from build123d import *

# Parameters (mm, degrees)
SWEEP1_START       = -3.175
SWEEP1_OUTLINE_W   = 31.75
SWEEP1_OUTLINE_H   = 57.15
SWEEP1_OUTLINE_W_2 = 19.05
SWEEP1_OUTLINE_H_2 = 44.45
SWEEP1_DEPTH       = 6.35
FILLET1_R          = 10
FILLET2_R          = 10


# Read off the part's stored shape, not the designer's step: Sweep1
with BuildPart() as part:
    # Sweep1 outline → Sweep1 (new body)
    with BuildSketch(Plane.XY.offset(SWEEP1_START)):
        with Locations((12.7, 25.4)):
            Rectangle(SWEEP1_OUTLINE_W, SWEEP1_OUTLINE_H)
        with Locations((12.7, 25.4)):
            Rectangle(SWEEP1_OUTLINE_W_2, SWEEP1_OUTLINE_H_2, mode=Mode.SUBTRACT)
    extrude(amount=SWEEP1_DEPTH)

    # Fillet1
    # the kernel refuses this fillet: 10 mm, written as the material it adds along each edge
    with BuildSketch(Plane(origin=(3.175, 3.175, -3.175), x_dir=(1, 0, 0), z_dir=(0, 0, 1)), Plane(origin=(22.225, 3.175, -3.175), x_dir=(0, 1, 0), z_dir=(0, 0, 1)), Plane(origin=(22.225, 47.625, -3.175), x_dir=(-1, 0, 0), z_dir=(0, 0, 1))) as fillet1_piece_1:
        with BuildLine():
            CenterArc((FILLET1_R, FILLET1_R), FILLET1_R, 180, 90)
            Line((0, FILLET1_R), (0, 0))
            Line((0, 0), (FILLET1_R, 0))
        make_face()
    extrude(amount=6.35)
    with BuildSketch(Plane(origin=(3.175, 47.625, -3.175), x_dir=(1, 0, 0), z_dir=(0, 0, 1))) as fillet1_piece_2:
        with BuildLine():
            CenterArc((FILLET1_R, -FILLET1_R), FILLET1_R, 90, 90)
            Line((0, -FILLET1_R), (0, 0))
            Line((0, 0), (FILLET1_R, 0))
        make_face()
    extrude(amount=6.35)

    # Fillet2
    fillet2_edges = [part.edges().sort_by_distance(p)[0] for p in [
        (28.575, -3.175, 0),
        (-3.175, 53.975, 0),
        (-3.175, -3.175, 0),
        (28.575, 53.975, 0),
    ]]
    fillet(fillet2_edges, radius=FILLET2_R)


solid = part.part
The model under review builds one solid part; all positions refer to its coordinate system, in mm. A direction names the side the tool comes from. Give positions to 0.01 mm unless a question says otherwise; leave off trailing zeros. Order: outer loops, then holes, each group sorted by start corner. A loop starts at its lowest first (then second) coordinate and runs counter-clockwise, first axis right, second up. Notation, with made-up numbers: M 46,-23 L 77,-23 A31 ccw 77,4 Z; hole C 89,23.25 d2. An arc over 180 degrees is marked long. Use one line per item in the form item = value. Start each with the question number.
Item 1: We need section D-D on y = 1. Give the boundary of the cut face in (x, z) (3 decimals), plus the area to 3 significant figures.
Item 2: We need section B-B on x = 14.5. Give the boundary of the cut face in (y, z) (3 decimals).
Item 3: The part is to be moulded in two halves that separate along Y. For faces 1 (the flat face through (22.225, 25, 0)), 2 (the cylindrical face through (25.57, -0.32, 0.04)), 3 (the flat face through (24, 26, 3.175)), say which applies: pulls with the +Y half, pulls with the -Y half, needs draft (parallel to the pull), parting line crosses it, or undercut.
Item 4: Insertion check: pin 1 Ø2 at (x, z) = (1, -2.5) entering from -Y. The pin has a flat end and moves straight along its axis. Give the tip position at first contact, or say it passes through.
Item 5: We need section C-C on z = 1. Give the boundary of the cut face in (x, y) (3 decimals), plus the area to 3 significant figures.
Item 6: To check wall thickness, follow line 1 along X through (y, z) = (19.5, 0.25) (3 decimals); line 2 along X through (y, z) = (5.5, 2.25); line 3 along Y through (x, z) = (8, 1.75) (3 decimals). State the ranges of each line that lie inside material, in increasing order. Write a range as from..to.
Item 7: For faces 4 (the cylindrical face through (25.57, 51.12, 0.04)), 5 (the cylindrical face through (5.865, 6.351, -0.044)), list the 3-axis set-ups (+Z, -Z, +X, -X, +Y, -Y) from which the entire face can be reached by the end or side of a thin tool; tool diameter is ignored.
Item 8: We need section A-A on y = 33. Give the boundary of the cut face in (x, z) (3 decimals), plus the area to 3 significant figures.
Completed:
q1.outline = M -1.303,-3.175 L 26.703,-3.175 L 26.703,3.175 L -1.303,3.175 Z
q1.area = 178 mm²
q2.outline = M -3.175,-3.175 L 3.437,-3.175 L 3.437,3.175 L -3.175,3.175 Z; M 47.363,-3.175 L 53.975,-3.175 L 53.975,3.175 L 47.363,3.175 Z
q3.face_1 = undercut
q3.face_2 = pulls with the -Y half
q3.face_3 = needs draft
q4.pin_1 = -1.93
q5.outline = M -3.175,6.825 A10 ccw 6.825,-3.175 L 18.575,-3.175 A10 ccw 28.575,6.825 L 28.575,43.975 A10 ccw 18.575,53.975 L 6.825,53.975 A10 ccw -3.175,43.975 Z; hole M 3.175,13.175 A10 ccw 12.7,3.186 A10 ccw 22.225,13.175 L 22.225,37.625 A10 ccw 12.7,47.614 A10 ccw 3.175,37.625 Z
q5.area = 968 mm²
q6.line_1 = -3.175..3.175, 22.225..28.575
q6.line_2 = -3.09..6.76, 18.64..28.49
q6.line_3 = -3.175..4.618, 46.182..53.975
q7.face_4 = +Z, -Z, +X, +Y
q7.face_5 = +Z, -Z
q8.outline = M -3.175,-3.175 L 3.175,-3.175 L 3.175,3.175 L -3.175,3.175 Z; M 22.225,-3.175 L 28.575,-3.175 L 28.575,3.175 L 22.225,3.175 Z
q8.area = 80.6 mm²
